The model under review builds one solid part; all positions refer to its coordinate system, in mm. A direction names the side the tool comes from. Give positions to 0.01 mm unless a question says otherwise; leave off trailing zeros. Order: outer loops, then holes, each group sorted by start corner. A loop starts at its lowest first (then second) coordinate and runs counter-clockwise, first axis right, second up. Notation, with made-up numbers: (-8.5, 62) - (40.5, 62) arc R26 cw to (40.5, 84) - close; hole circle Ø11 at (60, 49). An arc over 180 degrees is marked (long way). Use CSV: the item, a comma, the result in double quotes.
```python
from build123d import *

# Parameters (mm, degrees)
F0_R     = 3.2639
F0_R_2   = 3.37312
F0_W     = 50
F0_H     = 50
F1_DEPTH = 30
F2_R     = 12.7
F3_R     = 19.05
F4_R     = 3.37312
F5_DEPTH = 7.62
F6_R     = 4.9022
F7_DEPTH = 175.001


with BuildPart() as f1:
    # F0 (on Top) → F1 (new body)
    with BuildSketch(Plane.XY):
        Polygon((-100, -137.5), (-50, -137.5), (-50, -77.5), (-25, 17.5), (-25, 57.5), (25, 57.5), (25, 17.5), (50, -77.5), (50, -137.5), (100, -137.5), (100, -77.5), (75, 17.5), (75, 137.5), (-75, 137.5), (-75, 17.5), (-100, -77.5), align=None)
        with Locations((-87.5, -122.5)):
            Circle(F0_R, mode=Mode.SUBTRACT)
        with Locations((-62.5, -122.5)):
            Circle(F0_R, mode=Mode.SUBTRACT)
        with Locations((62.5, -122.5)):
            Circle(F0_R, mode=Mode.SUBTRACT)
        with Locations((87.5, -122.5)):
            Circle(F0_R, mode=Mode.SUBTRACT)
        with Locations((-40, 112.5)):
            Circle(F0_R_2, mode=Mode.SUBTRACT)
        with Locations((0, 97.5)):
            Rectangle(F0_W, F0_H, mode=Mode.SUBTRACT)
        with Locations((40, 112.5)):
            Circle(F0_R_2, mode=Mode.SUBTRACT)
        with Locations((-40, 112.5)):
            Circle(F0_R_2)
        with Locations((40, 112.5)):
            Circle(F0_R_2)
    extrude(amount=F1_DEPTH)

    # F2
    f2_edges = [f1.edges().sort_by_distance(p)[0] for p in [
        (-25, 122.5, 15),
        (25, 122.5, 15),
        (25, 72.5, 15),
        (-25, 72.5, 15),
        (-25, 57.5, 15),
        (25, 57.5, 15),
        (50, -77.5, 15),
        (-50, -77.5, 15),
        (-75, 17.5, 15),
        (75, 17.5, 15),
    ]]
    fillet(f2_edges, radius=F2_R)

    # F3
    f3_edges = [f1.edges().sort_by_distance(p)[0] for p in [
        (-100, -77.5, 15),
        (-75, 137.5, 15),
        (75, 137.5, 15),
        (100, -77.5, 15),
        (25, 17.5, 15),
        (-25, 17.5, 15),
    ]]
    fillet(f3_edges, radius=F3_R)

    # F4 (on face) → F5 (cut)
    with BuildSketch(Plane.XY.offset(30)):
        with Locations((-40, 112.5)):
            Circle(F4_R)
        with Locations((40, 112.5)):
            Circle(F4_R)
    extrude(amount=-F5_DEPTH, mode=Mode.SUBTRACT)

    # F6 (on face) → F7 (cut, through all)
    with BuildSketch(Plane(origin=(-75, 0, 0), x_dir=(0, -1, 0), z_dir=(-1, 0, 0))):
        with Locations((-97.5, 15)):
            Circle(F6_R)
    extrude(amount=-F7_DEPTH, mode=Mode.SUBTRACT)


solid = f1.part
```
Item 1: Clearance check with flat-ended pins moving along their axes: pin 1 (12 mm diameter, centred on y = 23.5, z = 4.5, fed in from +X); pin 2 (6 mm diameter, centred on y = 47.5, z = 16, fed in from -X); pin 3 (6 mm diameter, centred on x = -87.5, y = -122.5, fed in from +Z); pin 4 (5 mm diameter, centred on y = -45.5, z = 17.5, fed in from -X). State where each tip first meets the part, or that it passes through.
Results list:
pin 1,"stops at x = 75.11"
pin 2,"stops at x = -75"
pin 3,"passes through"
pin 4,"stops at x = -92.24"
Item 2: Take a section at A-A, the plane y = 97.5. Give the boundary of the cut face in (x, z).
Results list:
outline,"(-75, 0) - (-25, 0) - (-25, 10.1) - (-75, 10.1) - close; (-75, 19.9) - (-25, 19.9) - (-25, 30) - (-75, 30) - close; (25, 0) - (75, 0) - (75, 10.1) - (25, 10.1) - close; (25, 19.9) - (75, 19.9) - (75, 30) - (25, 30) - close"
Item 3: Take a section at D-D, the plane x = -40. Give the boundary of the cut face in (y, z), and give its area (3 significant figures).
Results list:
outline,"(-39.5, 0) - (137.5, 0) - (137.5, 30) - (115.87, 30) - (115.87, 22.38) - (109.13, 22.38) - (109.13, 30) - (-39.5, 30) - close; hole circle Ø9.8 at (97.5, 15)"
area,"5,180 mm2"
Item 4: Mouldability with a two-part tool opening along Z and no side actions: class faces 1 (the face through (0, 72.5, 15)), 2 (the face through (-46, 2, 30)), 3 (the face through (-50.4, 102.4, 15.2)) as pulls with the +Z half, pulls with the -Z half, needs draft (parallel to the pull), parting line crosses it, or undercut.
Results list:
face 1,"needs draft"
face 2,"pulls with the +Z half"
face 3,"undercut"
Item 5: Tool access review of faces 4 (the face through (40, 113, 22.38)), 5 (the face through (0, 57.5, 15)), 6 (the face through (1, 137.5, 15)), 7 (the face through (-25, 92, 15)): name each direction out of +Z, -Z, +X, -X, +Y, -Y from which nothing blocks a thin tool from reaching the whole face with its end or side.
Results list:
face 4,"+Z"
face 5,"+Z, -Z, -Y"
face 6,"+Z, -Z, +X, -X, +Y"
face 7,"+Z, -Z"
Item 6: Take a section at C-C, the plane z = 15. State how many separate pieces and enclosed holes the cut face has, and give its area (3 significant figures).
Results list:
separate pieces,"2"
enclosed holes,"4"
area,"27,900 mm2"
Item 7: Wall thickness on L1, parallel to X at y = 44.5, z = 16.75; L2, parallel to Y at x = 6, z = 28; L3, parallel to Z at x = -46, y = 97.5: over which ranges is each line inside the solid? List them lowest first.
Results list:
L1,"x = -75 to -25, 25 to 75"
L2,"y = 57.5 to 72.5, 122.5 to 137.5"
L3,"z = 0 to 10.1, 19.9 to 30"
Item 8: Take a section at B-B, the plane x = 87.5. Give the boundary of the cut face in (y, z).
Results list:
outline,"(-137.5, 0) - (-125.76, 0) - (-125.76, 30) - (-137.5, 30) - close; (-119.24, 0) - (-30, 0) - (-30, 30) - (-119.24, 30) - close"
